from build123d import *

# Parameters (mm, degrees)
F3_DEPTH = 50.8
F4_R     = 31.75
F5_DEPTH = 50.8
F5_TAPER = -10


# Not quite as in the source:
# - the program builds the solid bodies; features that only make, move or delete a surface that nothing else refers to are left out


with BuildPart() as f3:
    # F2 (on face) → F3 (new body)
    with BuildSketch(Plane.XY.offset(-76.2)):
        with BuildLine():
            Line((6.0835533113, 3.175), (18.7835533113, 3.175))
            ThreePointArc((18.7835533113, 3.175), (-19.05, 0), (18.7835533113, -3.175))
            Line((18.7835533113, -3.175), (6.0835533113, -3.175))
            Line((6.0835533113, -3.175), (6.0835533113, 3.175))
        make_face()
    extrude(amount=-F3_DEPTH)

    # F4 (on face) → F5 (join)
    with BuildSketch(Plane(origin=(0, 0, -127), x_dir=(1, 0, 0), z_dir=(0, 0, -1))):
        Circle(F4_R)
    extrude(amount=F5_DEPTH, taper=F5_TAPER)


solid = f3.part
The listing builds one solid part. Answer for the finished solid, in the listing's coordinates (mm). A direction names the side the tool comes from. Coordinates: 2 decimals unless noted, no trailing zeros. Loops run counter-clockwise (first coordinate to the right, second up) from the corner with the lowest first, then second, coordinate; pieces in that order, holes last.
1) Find section A-A on x = 0. Write down the section's boundary in (y, z).
2) A tool of negligible diameter and unlimited length cuts with its end or side. For faces 4 (the face through (-1, -1, -177.8)), 5 (the face through (13, -3.175, -101)), 6 (the face through (-19.033, 0.793, -101.244)), from which of +Z, -Z, +X, -X, +Y, -Y can it reach the whole face along a straight path? Write none if from no direction.
3) Flat-ended cylindrical pins translate along their axes: pin 1 Ø5 at (x, z) = (-1, -88.5) entering from -Y; pin 2 Ø8 at (x, z) = (-21.5, -121.5) entering from +Y; pin 3 Ø1 at (x, z) = (15, -165.5) entering from +Y. Find the tip coordinate at first contact, or state that the pin passes through.
4) Determine the mould class of faces 1 (the face through (33.666, -10.602, -147.111)), 2 (the face through (0, 0, -76.2)), 3 (the face through (12, 3.175, -101)) for opening direction Y: pulls with the +Y half, pulls with the -Y half, needs draft (parallel to the pull), parting line crosses it, or undercut.
5) Find section C-C on z = -135. Write down the section's boundary in (x, y).
6) Find the intervals of material crossed by L1, parallel to Z at x = -22.5, y = -7; L2, parallel to X at y = 0.5, z = -121.5; L3, parallel to X at y = -17.5, z = -153, in increasing order.
7) Find section B-B on z = -91. Write down the section's boundary in (x, y) (3 decimals).
8) Find section D-D on z = -166. Write down the section's boundary in (x, y).
Values:
1. outline: (-40.71, -177.8) - (40.71, -177.8) - (31.75, -127) - (19.05, -127) - (19.05, -76.2) - (-19.05, -76.2) - (-19.05, -127) - (-31.75, -127) - close
2. face 4: -Z, +X, -X, +Y, -Y
2. face 5: +Z, +X
2. face 6: +Z
3. pin 1: stops at y = -19.05
3. pin 2: stops at y = 7.53
3. pin 3: stops at y = 35.73
4. face 1: parting line crosses it
4. face 2: needs draft
4. face 3: undercut
5. outline: circle Ø66.32 at (0, 0)
6. L1: z = -177.8 to -127
6. L2: x = -19.04 to 6.08
6. L3: x = -31.84 to 31.84
7. outline: (6.084, -3.175) - (6.084, 3.175) - (18.784, 3.175) arc R19.05 ccw (long way) to (18.784, -3.175) - close
8. outline: circle Ø77.25 at (0, 0)
